```python
from build123d import *

# Parameters (mm, degrees)
F0_R     = 1
F1_DEPTH = 8
F0_W     = 23
F0_H     = 6
F2_DEPTH = 40
F4_START = 35
F3_W     = 8
F3_H     = 40
F4_DEPTH = 5


with BuildPart() as f1:
    # F0 (on Top) → F1 (new body)
    with BuildSketch(Plane.XY):
        Polygon((-11.5, 1.7857142857), (-11.5, 7.7857142857), (-16.5, 7.7857142857), (-16.5, -10.2142857143), (-11.5, -10.2142857143), align=None)
        with Locations((-14, -4.7142857143)):
            Circle(F0_R, mode=Mode.SUBTRACT)
    extrude(amount=F1_DEPTH)



with BuildPart() as f1b:
    # F0 (on Top) → F1, piece 2 (new body)
    with BuildSketch(Plane.XY):
        Polygon((16.5, 7.7857142857), (11.5, 7.7857142857), (11.5, 1.7857142857), (11.5, -10.2142857143), (16.5, -10.2142857143), align=None)
        with Locations((14, -4.7142857143)):
            Circle(F0_R, mode=Mode.SUBTRACT)
    extrude(amount=F1_DEPTH)


with BuildPart() as f1_1:
    add(f1.part)

    add(f1b.part)  # F2 merges F1b
    # F0 (on Top) → F2 (join)
    with BuildSketch(Plane.XY):
        with Locations((0, 4.7857142857)):
            Rectangle(F0_W, F0_H)
    extrude(amount=F2_DEPTH)

    # F3 (on Top) → F4 (join)
    with BuildSketch(Plane.XY.offset(F4_START)):
        with Locations((-7.5, 27.7857142857)):
            Rectangle(F3_W, F3_H)
        with Locations((7.5, 27.7857142857)):
            Rectangle(F3_W, F3_H)
        with Locations((0, -18.2142857143)):
            Rectangle(F3_W, F3_H)
    extrude(amount=F4_DEPTH)


solid = f1_1.part
```
For this review, take the finished solid that the model builds, in its own axes (mm). A direction names the side the tool comes from. Give positions to 0.01 mm unless a question says otherwise; leave off trailing zeros. Write each loop counter-clockwise with the first axis right and the second up, starting at its lowest first coordinate (ties: lowest second). Pieces come first, ordered by that corner, then holes. Notation, with made-up numbers: M 7.5,34.25 L 62.5,34.25 A28 ccw 62.5,60.25 Z; hole C 25.5,65.5 d11. An arc over 180 degrees is marked long. Answer as a JSON object with one key per item and string values. Group by question number.
Item 1: Consider section B-B on y = 41. Write out the cut boundary in (x, z).
Item 2: Draft analysis for pull direction X (two halves, no side actions). For faces 6 (the flat face through (3.5, 28, 37)), 7 (the flat face through (5, 15, 40)), 8 (the flat face through (16.5, -1, 4)), state which applies: +X half, -X half, draft (parallel to the pull), parting line (faces both ways), or undercut.
Item 3: Consider section D-D on z = 5.5. Write out the cut boundary in (x, y).
Item 4: For pin 1 Ø2.5 at (y, z) = (26.5, 36.5) entering from +X; pin 2 Ø1.2 at (x, y) = (14, -4.71) entering from -Z; pin 3 Ø9 at (x, y) = (9, 27.5) entering from -Z; pin 4 Ø4 at (x, y) = (-14.5, -1.5) entering from +Z, all flat-tipped, find the tip position at first contact; note any pin that passes through.
Item 5: Tool access review of faces 1 (the flat face through (-11.5, 16, 36)), 2 (the flat face through (4, -18, 37)), 3 (the flat face through (11.5, 16, 36)), 4 (the flat face through (0, -18, 35)), 5 (the flat face through (-11.5, -4, 4)): name each direction out of +Z, -Z, +X, -X, +Y, -Y from which nothing blocks a thin tool from reaching the whole face with its end or side.
Item 6: Consider section C-C on z = 37. Write out the cut boundary in (x, y).
Item 7: For probe 1 along Z at (x, y) = (-12, 6.5); probe 2 along Y at (x, z) = (14, 4.5); probe 3 along Z at (x, y) = (-10, 13.5), list the stretches that pass through material, from the lowest coordinate up. Write a range as [from, to].
Item 8: Consider section A-A on x = 14. Write out the cut boundary in (y, z).
Check result:
{
 "1": {"outline": "M -11.5,35 L -3.5,35 L -3.5,40 L -11.5,40 Z; M 3.5,35 L 11.5,35 L 11.5,40 L 3.5,40 Z"},
 "2": {"face 6": "undercut", "face 7": "draft", "face 8": "+X half"},
 "3": {"outline": "M -16.5,-10.21 L -11.5,-10.21 L -11.5,1.79 L 11.5,1.79 L 11.5,-10.21 L 16.5,-10.21 L 16.5,7.79 L -16.5,7.79 Z; hole C -14,-4.71 d2; hole C 14,-4.71 d2"},
 "4": {"pin 1": "stops at x = 11.5", "pin 2": "passes through", "pin 3": "stops at z = 35", "pin 4": "stops at z = 8"},
 "5": {"face 1": "+Z, -X, +Y, -Y", "face 2": "+Z, -Z, +X, -Y", "face 3": "+Z, +X, +Y, -Y", "face 4": "-Z, +X, -X, -Y", "face 5": "+Z, -Z, -Y"},
 "6": {"outline": "M -11.5,1.79 L -4,1.79 L -4,-38.21 L 4,-38.21 L 4,1.79 L 11.5,1.79 L 11.5,47.79 L 3.5,47.79 L 3.5,7.79 L -3.5,7.79 L -3.5,47.79 L -11.5,47.79 Z"},
 "7": {"probe 1": "z = [0, 8]", "probe 2": "y = [-10.21, -5.71], [-3.71, 7.79]", "probe 3": "z = [35, 40]"},
 "8": {"outline": "M -10.21,0 L -5.71,0 L -5.71,8 L -10.21,8 Z; M -3.71,0 L 7.79,0 L 7.79,8 L -3.71,8 Z"}
}
